Drawing for the job (mm, zero at the part's lowest x, y, z). Coordinates: 2 decimals unless noted, no trailing zeros. Write each loop counter-clockwise with the first axis right and the second up, starting at its lowest first coordinate (ties: lowest second). Pieces come first, ordered by that corner, then holes. Notation, with made-up numbers: (14, -4.5) -> (21, -4.5) arc R22 ccw to (21, 7.5) -> close; hole circle Ø9 at (-20.5, -5.5). An arc over 180 degrees is marked (long way). Answer as CSV lines item,"result".
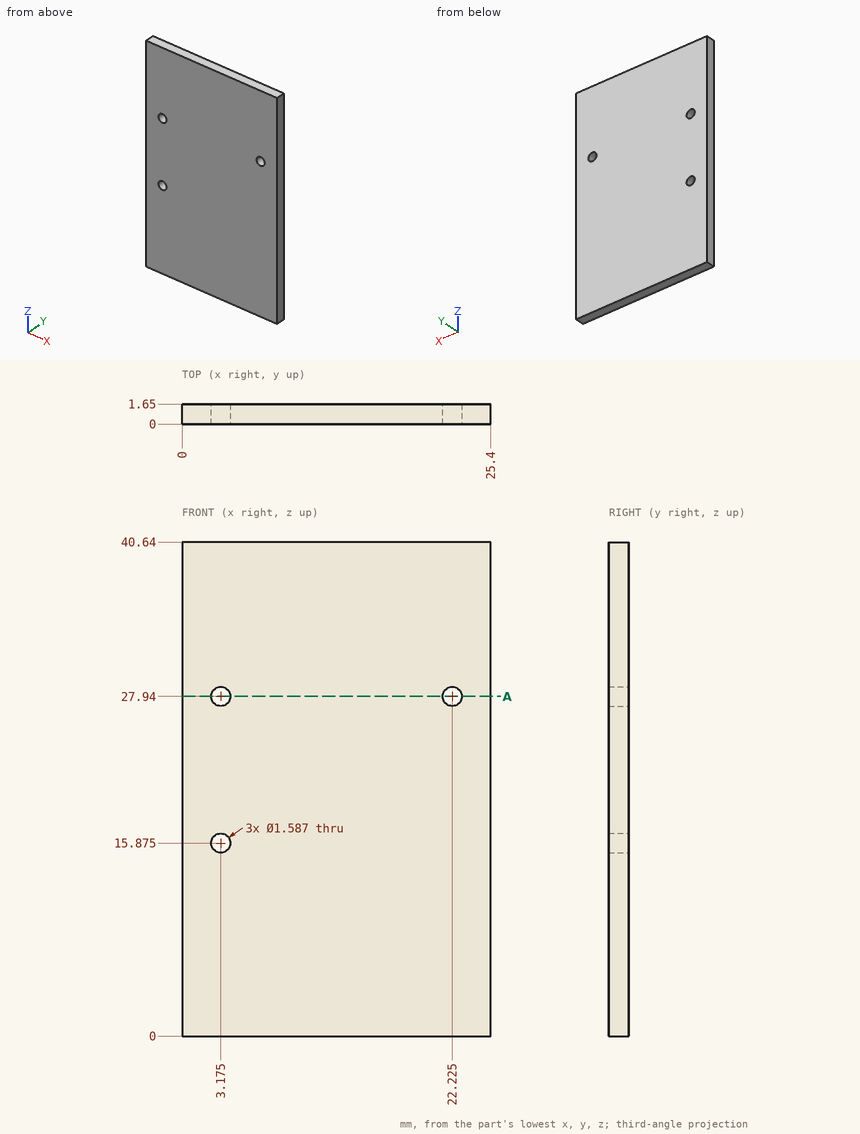
Item 1: Wall check: line 1 (X direction, y = 0.35, z = 27.94); line 2 (Z direction, x = 22, y = 1.05); line 3 (X direction, y = 1.6, z = 15.5) (1 decimal). Give the ranges that are in metal, low to high. Write a range as from..to.
Answer below:
line 1,"x = 0..2.38, 3.97..21.43, 23.02..25.4"
line 2,"z = 0..27.18, 28.7..40.64"
line 3,"x = 0..2.5, 3.9..25.4"
Item 2: Saw through at A-A on z = 27.94. Give the cut face in (x, y).
Answer below:
outline,"(0, 0) -> (2.38, 0) -> (2.38, 1.65) -> (0, 1.65) -> close; (3.97, 0) -> (21.43, 0) -> (21.43, 1.65) -> (3.97, 1.65) -> close; (23.02, 0) -> (25.4, 0) -> (25.4, 1.65) -> (23.02, 1.65) -> close"
Item 3: Flat gauge pin, fed straight in: pin 1 (1 mm diameter, centred on x = 3.175, z = 27.94, fed in from -Y). Where does the tip first touch, or does it go through?
Answer below:
pin 1,"passes through"
